Autodesk Inventor part; units mm, degrees
ref_plane "YZ Plane" through (0, 0, 0) normal (1, 0, 0) x (0, 1, 0)
ref_plane "XZ Plane" through (0, 0, 0) normal (0, 1, 0) x (-1, 0, 0)
ref_plane "XY Plane" through (0, 0, 0) normal (0, 0, 1) x (1, 0, 0)
sketch "Sketch1" plane through (0, 0, 0) normal (0, 1, 0) x (-1, 0, 0)
  line L0 (150, 70) -> (-150, 70)
  line L1 (-150, 70) -> (-150, 0)
  line L2 (-150, 0) -> (150, 0)
  line L3 (150, 0) -> (150, 70)
  line L4 (150, 0) -> (0, -20)
  line L5 (0, -20) -> (-150, 0)
  point P0 (0, 0)
  point P1 (0, 0)
  dimension "d0" = 300
  dimension "d1" = 70
  dimension "d2" = 20
extrude "Extrusion1" add sketch "Sketch1" along normal blind 600
sketch "Sketch2" plane through (-150, 0, 70) normal (0, 0, 1) x (1, 0, 0)
  line L0 (0, 0) -> (300, 0)
  line L1 (300, 0) -> (300, 600)
  line L2 (0, 600) -> (300, 600)
  line L3 (0, 0) -> (0, 600)
  ellipse E0 centre (150, 370) end of major axis (0, 370) minor radius 200
  line L4 (0, 370) -> (150, 570)
  line L5 (150, 570) -> (300, 370)
  point P0 (150, 0)
  point P1 (150, 600)
  dimension "d7" = 200
  dimension "d5" = 370
extrude "Extrusion2" cut sketch "Sketch2" against normal through all contours L3 L2 L1 E0 | E0 L4 | L5 E0
sketch "Sketch3" plane through (-150, 0, 0) normal (-1, 0, 0) x (0, 0, 1)
  line L0 (70, 570) -> (-20, 570)
  line L1 (-20, 0) -> (-20, 570)
  line L2 (30, 570) -> (-20, 236.6667)
  point P0 (0, 0)
  point P1 (0, 370)
  dimension "d11" = 40
extrude "Extrusion3" cut sketch "Sketch3" against normal through all
shell "Shell2" thickness 4 removed faces 1 at (50, 246.6667, 70)
properties part number "Generalcraftshape1"
Verification items for the finished model (mm, model axes). A direction names the side the tool comes from. Coordinates: 2 decimals unless noted, no trailing zeros. Write each loop counter-clockwise with the first axis right and the second up, starting at its lowest first coordinate (ties: lowest second). Pieces come first, ordered by that corner, then holes. Notation, with made-up numbers: (-40, 23.5) - (-19, 23.5) arc R10 cw to (-19, 35.5) - close; hole circle Ø7 at (37.5, -39). An arc over 180 degrees is marked (long way). One line per question, with ' | ' between items. Start each with the question number.
1. Section check C-C (x = -90.5). Enter the section's corners in (y, z), plus the area to 3 significant figures.
2. Section check B-B (y = 163). Enter the section's corners in (x, z), plus the area to 3 significant figures.
3. Section check A-A (z = 46.5). Enter the section's corners in (x, y).
4. Access from +Z, -Z, +X, -X, +Y, -Y to the whole of each face (thin tool, end or side, straight path). Record for faces 1 (the flat face through (-76.05, 468.6, 43.27)), 2 (the flat face through (-2.044, 402.256, 8.883)).
5. Draft check along Y on faces 3 (the flat face through (-74.022, 142.39, -6.095)), 4 (the flat face through (-76.05, 141.3, -9.86)), 5 (the flat face through (73.95, 471.4, 43.27)). Enter one of: released by +Y, released by -Y, zero draft, split by the parting line, or undercut.
6. Section check D-D (z = 19.5). Enter the section's corners in (x, y) (3 decimals).
7. Material ranges on line 1 along X through (y, z) = (80, 61.5); line 2 along X through (y, z) = (487, 32.5); line 3 along Y through (x, z) = (-1.5, 61), recorded low to high.
8. Gauge pin test, flat ends, axial feed: P1, Ø6, axis at x = 56.5, y = 412.5, coming from the -Z side (3 decimals); P2, Ø5, axis at x = 71.5, y = 189.5, coming from the +Z side; P3, Ø10, axis at y = 384, z = 20, coming from the -X side. Record the tip position at first contact, or that the pin passes through.
Computed values:
1) outline: (0, -7.93) - (317.11, -7.93) - (449.33, 11.9) - (449.33, 70) - (442.67, 70) - (442.67, 14.94) - (317.05, -3.9) - (4, -3.9) - (4, 70) - (0, 70) - close | area: 2,470 mm²
2) outline: (-150, 0) - (0, -20) - (150, 0) - (150, 70) - (146, 70) - (146, 3.5) - (0, -15.96) - (-146, 3.5) - (-146, 70) - (-150, 70) - close | area: 1,740 mm²
3) outline: (-150, 0) - (150, 0) - (150, 370) - (0, 570) - (-150, 370) - close; hole (-146, 4) - (146, 4) - (146, 368.67) - (0, 563.33) - (-146, 368.67) - close
4) face 1: +Z, -Z, -X, +Y | face 2: +Z
5) face 3: undercut | face 4: zero draft | face 5: released by +Y
6) outline: (-150, 0) - (150, 0) - (150, 370) - (52.5, 500) - (-52.5, 500) - (-150, 370) - close; hole (-146, 4) - (146, 4) - (146, 368.667) - (67.724, 473.035) - (-67.724, 473.035) - (-146, 368.667) - close
7) line 1: -150 to -146, 146 to 150 | line 2: -62.25 to -57.25, 57.25 to 62.25 | line 3: 0 to 4, 561.33 to 568
8) P1: z = 5.925 | P2: z = -6.1 | P3: x = -143.25
